from build123d import *

# Parameters (mm, degrees)
F1_DEPTH = 25.4
F3_DEPTH = 25.4
F5_DEPTH = 25.4
F6_W     = 17.318182
F6_H     = 16.51
F7_DEPTH = 7.366


with BuildPart() as f1:
    # F0 (on Front) → F1 (new body)
    with BuildSketch(Plane.XZ):
        Polygon((0, 0), (31.634543, 0), (31.634543, 8.428182), (10.39091, 8.428182), (10.39091, 46.990003), (0, 46.990003), align=None)
    extrude(amount=F1_DEPTH)

    # F2 (on face) → F3 (cut)
    with BuildSketch(Plane.XY.offset(8.428182)):
        with BuildLine():
            ThreePointArc((24.34968, -0.09495), (31.634543, -12.7), (24.34968, -25.30505))
            ThreePointArc((24.34968, -25.30505), (46.19327, -12.7), (24.34968, -0.09495))
        make_face()
    extrude(amount=-F3_DEPTH, mode=Mode.SUBTRACT)

    # F4 (on face) → F5 (cut)
    with BuildSketch(Plane.YZ.offset(10.39091)):
        with BuildLine():
            Line((-17.84547, 27.61518), (-17.845491, 28.49549))
            ThreePointArc((-17.845491, 28.49549), (-17.864271, 28.055334), (-17.84547, 27.61518))
        make_face()
        with BuildLine():
            Line((-17.845925, 46.990003), (-17.845491, 28.49549))
            Line((-17.845491, 28.49549), (-17.84547, 27.61518))
            ThreePointArc((-17.84547, 27.61518), (-12.918515, 22.895384), (-7.609436, 27.180831))
            Line((-7.609436, 27.180831), (-7.609436, 28.93008))
            Line((-7.609436, 28.93008), (-7.609436, 46.990003))
            Line((-7.609436, 46.990003), (-17.845925, 46.990003))
        make_face()
        with BuildLine():
            Line((-7.609436, 28.93008), (-7.609436, 27.180831))
            ThreePointArc((-7.609436, 27.180831), (-7.534841, 28.055456), (-7.609436, 28.93008))
        make_face()
    extrude(amount=-F5_DEPTH, mode=Mode.SUBTRACT)

    # F6 (on face) → F7 (cut)
    with BuildSketch(Plane(origin=(0, 0, 0), x_dir=(-1, 0, 0), z_dir=(0, 1, 0))):
        with Locations((-8.659091, 8.255)):
            Rectangle(F6_W, F6_H)
    extrude(amount=-F7_DEPTH, mode=Mode.SUBTRACT)


solid = f1.part
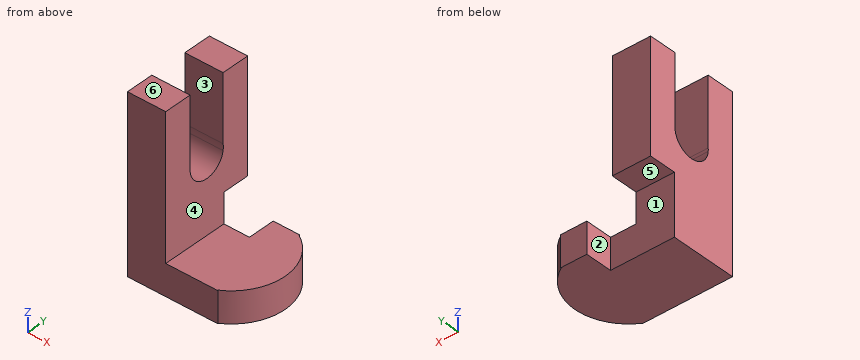
Can you work these out from the model? Positions are in its coordinate system, mm. Face numbers are marked on the shaded views. A direction names the side the tool comes from. Give positions to 0.01 mm unless a question says otherwise; leave off trailing zeros. Order: outer loops, then holes, each group sorted by start corner. A loop starts at its lowest first (then second) coordinate and runs counter-clockwise, first axis right, second up. Notation, with made-up numbers: M 45.5,2.25 L 53.5,2.25 A21 ccw 53.5,33.25 Z; hole C 38.5,-18 d10. An arc over 180 degrees is marked long. Use one line per item in the form item = value.
Item 1: Will these pins go through, and if not, where does the flat tip stop? pin 1 Ø1 at (x, y) = (21.5, -18.5) entering from +Z; pin 2 Ø6 at (x, z) = (12, 10) entering from +Y; pin 3 Ø8 at (y, z) = (-3, 3) entering from -X.
Values follow:
pin_1 = 8.43
pin_2 = -7.37
pin_3 = 17.32
Item 2: If we section it at A-A, the plane x = 7.5: Write out the boundary of the cut face in (y, z).
Values follow:
outline = M -25.4,0 L -7.37,0 L -7.37,16.51 L 0,16.51 L 0,46.99 L -7.61,46.99 L -7.61,28.93 A5.16 cw -7.61,27.18 A5.16 cw -17.85,27.62 A5.16 cw -17.85,28.5 L -17.85,46.99 L -25.4,46.99 Z
Item 3: For the marked faces 4, 5 and 6, which set-ups out of +Z, -Z, +X, -X, +Y, -Y let a thin tool reach every point of the face, with its end or its side?
Values follow:
face_4 = +Z, +X, +Y, -Y
face_5 = -Z, +X, -X, +Y
face_6 = +Z, +X, -X, +Y, -Y
Item 4: If we section it at C-C, the plane y = -2.75: Write out the boundary of the cut face in (x, z), and give its area (3 significant figures).
Values follow:
outline = M 0,16.51 L 10.39,16.51 L 10.39,46.99 L 0,46.99 Z; M 17.32,0 L 27.7,0 L 27.7,8.43 L 17.32,8.43 Z
area = 404 mm^2
Item 5: Thinking about a two-plate mould opening in Y: for the marked faces 1, 2 and 3, which applies, pulls with the +Y half, pulls with the -Y half, needs draft (parallel to the pull), parting line crosses it, or undercut?
Values follow:
face_1 = pulls with the +Y half
face_2 = needs draft
face_3 = undercut
Item 6: If I drill on line 1 along Y through (x, z) = (5.5, 39); line 2 along Z through (x, y) = (22.5, -16.5); line 3 along Y through (x, z) = (13.5, 5), over which ranges is the centre line in solid material (lowest first)? Write a range as [from, to].
Values follow:
line_1 = [-25.4, -17.85], [-7.61, 0]
line_2 = [0, 8.43]
line_3 = [-25.4, -7.37]
Item 7: If we section it at D-D, the plane z = 5.5: Write out the boundary of the cut face in (x, y).
Values follow:
outline = M 0,-25.4 L 24.52,-25.4 A14.56 cw 24.35,-25.31 A14.55 ccw 24.35,-0.09 A14.56 cw 24.52,0 L 17.32,0 L 17.32,-7.37 L 0,-7.37 Z
Item 8: If we section it at B-B, the plane z = 37: Write out the boundary of the cut face in (x, y).
Values follow:
outline = M 0,-25.4 L 10.39,-25.4 L 10.39,-17.85 L 0,-17.85 Z; M 0,-7.61 L 10.39,-7.61 L 10.39,0 L 0,0 Z
